Read the model definition and answer for the solid it produces. Units are mm, in the model's axes. Face numbers are marked on the shaded views. A direction names the side the tool comes from. Give positions to 0.01 mm unless a question says otherwise; leave off trailing zeros. Write each loop counter-clockwise with the first axis right and the second up, starting at its lowest first coordinate (ties: lowest second). Pieces come first, ordered by that corner, then holes. Notation, with made-up numbers: (-29.75, -34.75) -> (20.25, -34.75) arc R12 ccw to (20.25, -26.75) -> close; hole circle Ø6 at (-22.5, 62.5). An arc over 180 degrees is marked (long way). Use a Markdown table: item, result.
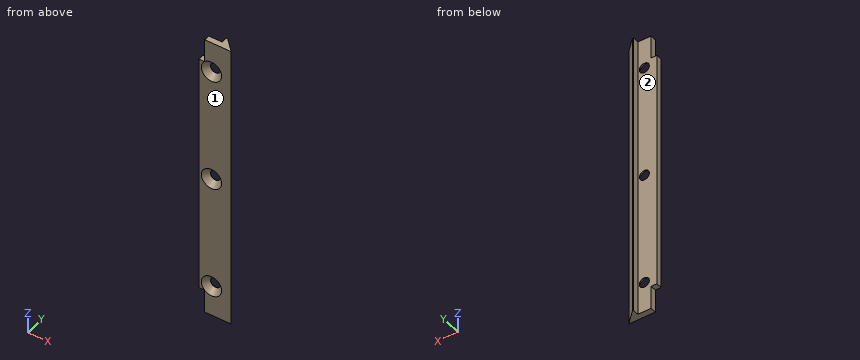
Autodesk Inventor part; units mm, degrees
ref_plane "YZ Plane" through (0, 0, 0) normal (1, 0, 0) x (0, 1, 0)
ref_plane "XZ Plane" through (0, 0, 0) normal (0, 1, 0) x (-1, 0, 0)
ref_plane "XY Plane" through (0, 0, 0) normal (0, 0, 1) x (1, 0, 0)
sketch "Szkic1" plane through (0, 0, 0) normal (0, 0, 1) x (1, 0, 0)
  line L0 (0, 0) -> (11, 0)
  line L1 (11, 0) -> (7, 4)
  line L2 (7, 4) -> (6.5, 4)
  line L3 (6.5, 4) -> (6.5, 2)
  line L4 (6.5, 2) -> (0, 2)
  line L5 (0, 2) -> (0, 0)
  dimension "d1" = 45
  dimension "d3" = 2
  dimension "d4" = 2
  dimension "d5" = 11
  dimension "d19" = 4.5
extrude "Wyciągnięcie proste1" add sketch "Szkic1" against normal blind 98
sketch "Szkic4" plane through (0, 0, 0) normal (0, -1, 0) x (1, 0, 0)
  line L0 (0, 0) -> (0, -98) construction
  line L1 (0, -49) -> (11, -49) construction
  line L2 (11, 0) -> (11, -98) construction
  line L3 (4.3, -10.4) -> (4.3, -49) construction
  line L4 (6.5, 0) -> (6.5, -98) construction
  point P0 (4.3, -87.6)
  dimension "d10" = 2.2
  dimension "d11" = 38.6
hole "Otwór1" at (4.3, 0, -10.4) at (4.3, 0, -49) at (4.3, 0, -87.6) direction (0, 1, 0) diameter 3.4 end through all countersink diameter 6.9 countersink angle 84.225
sketch "Szkic5" plane through (0, 2, 0) normal (0, 1, 0) x (1, 0, 0)
  line L0 (0, 0) -> (11, 0)
  line L1 (0, 0) -> (2, 0)
  line L2 (2, 0) -> (2, 7.9)
  line L3 (2, 7.9) -> (0, 7.9)
  line L4 (0, 7.9) -> (0, 0)
  line L5 (0, 0) -> (0, 98) construction
  line L6 (0, 49) -> (11, 49) construction
  line L7 (11, 0) -> (11, 98) construction
  line L8 (6.5, 0) -> (6.5, 98) construction
  line L9 (0, 98) -> (2, 98)
  line L10 (2, 98) -> (2, 90.1)
  line L11 (2, 90.1) -> (0, 90.1)
  line L12 (0, 90.1) -> (0, 98)
  dimension "d20" = 4.5
  dimension "d21" = 7.9
extrude "Wyciągnięcie proste2" cut sketch "Szkic5" against normal through all
properties part number "Plug"
Item 1: A cutting plane is placed at B-B (z = -87.6). Give the vertices of the cut face in (x, y).
Return value:
| item | result |
|---|---|
| outline | (0, 0) -> (0.85, 0) -> (2.6, 1.94) -> (2.6, 2) -> (0, 2) -> close; (6, 1.94) -> (7.75, 0) -> (11, 0) -> (7, 4) -> (6.5, 4) -> (6.5, 2) -> (6, 2) -> close |
Item 2: A cutting plane is placed at A-A (x = 4.3). Give the vertices of the cut face in (y, z), then the cut area to 3 significant figures.
Return value:
| item | result |
|---|---|
| outline | (0, -98) -> (2, -98) -> (2, -89.3) -> (1.94, -89.3) -> (0, -91.05) -> close; (0, -84.15) -> (1.94, -85.9) -> (2, -85.9) -> (2, -50.7) -> (1.94, -50.7) -> (0, -52.45) -> close; (0, -45.55) -> (1.94, -47.3) -> (2, -47.3) -> (2, -12.1) -> (1.94, -12.1) -> (0, -13.85) -> close; (0, -6.95) -> (1.94, -8.7) -> (2, -8.7) -> (2, 0) -> (0, 0) -> close |
| area | 165 mm^2 |
Item 3: A cutting plane is placed at C-C (z = -42.5). Give the vertices of the cut face in (x, y).
Return value:
| item | result |
|---|---|
| outline | (0, 0) -> (11, 0) -> (7, 4) -> (6.5, 4) -> (6.5, 2) -> (0, 2) -> close |
Item 4: A cutting plane is placed at D-D (x = 9). Give the vertices of the cut face in (y, z).
Return value:
| item | result |
|---|---|
| outline | (0, -98) -> (2, -98) -> (2, 0) -> (0, 0) -> close |
Item 5: Each of these flat-tipped pins is pushed along its axis until it touches: P1, Ø2, axis at x = 1.5, y = 1.5, coming from the +Z side; P2, Ø0.6, axis at y = 1, z = -4.5, coming from the -X side; P3, Ø1, axis at x = 4, z = -33.5, coming from the +Y side. Where does it stop, or does it pass through?
Return value:
| item | result |
|---|---|
| P1 | z = 0 |
| P2 | x = 2 |
| P3 | y = 2 |
Item 6: A tool of negligible diameter and unlimited length cuts with its end or side. For the marked faces 1 and 2, from which of +Z, -Z, +X, -X, +Y, -Y can it reach the whole face along a straight path? Write none if from no direction.
Return value:
| item | result |
|---|---|
| face 1 | +Z, -Z, +X, -X, -Y |
| face 2 | +Z, -Z, -X, +Y |
Item 7: Straight lines are drawn through the part: line 1 along Z through (x, y) = (4.3, 1.9); line 2 along Z through (x, y) = (6.75, 0.3); line 3 along Y through (x, z) = (6.25, -25). For each, find the intervals that lie inside material, in ascending order. Write a range as [from, to].
Return value:
| item | result |
|---|---|
| line 1 | [-98, -89.33], [-85.87, -50.73], [-47.27, -12.13], [-8.67, 0] |
| line 2 | [-98, -89.63], [-85.57, -51.03], [-46.97, -12.43], [-8.37, 0] |
| line 3 | [0, 2] |
